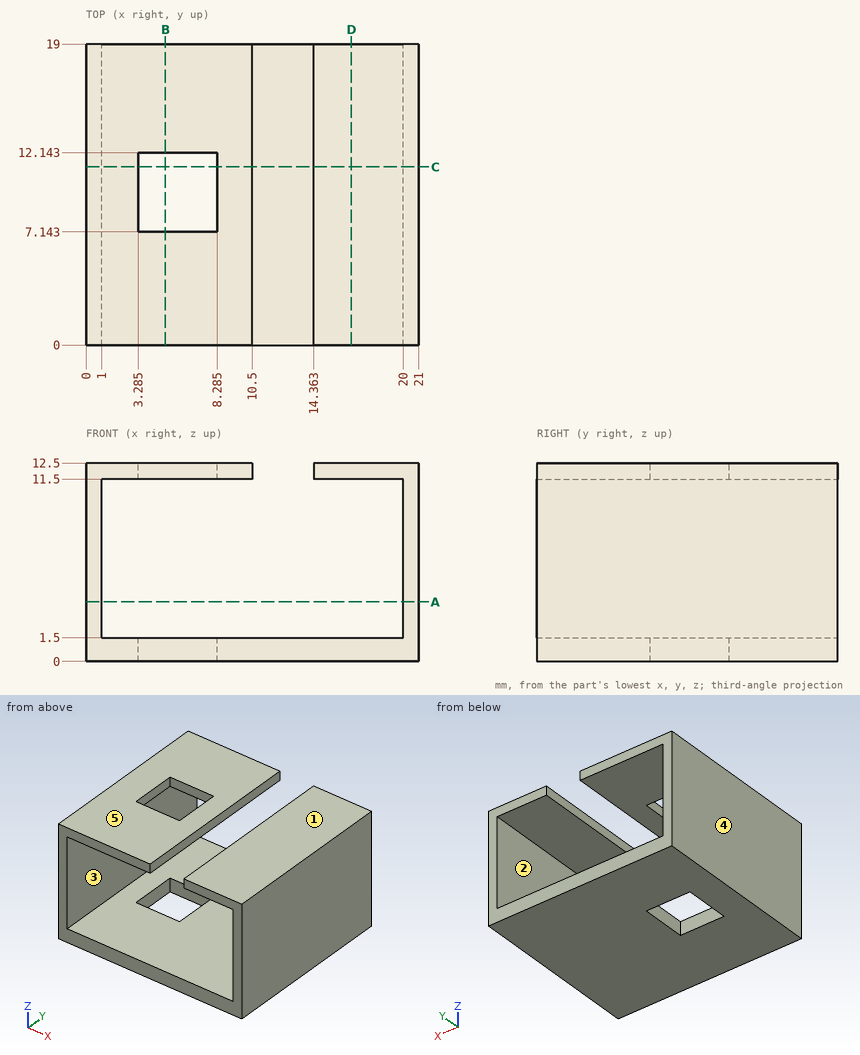
Source: three-view drawing plus pictorial views. Frame: mm from the lowest corner of the part. A direction names the side the tool comes from. Round coordinates to 2 decimals unless told otherwise and drop trailing zeros. Loops run counter-clockwise (first coordinate to the right, second up) from the corner with the lowest first, then second, coordinate; pieces in that order, holes last. Notation, with made-up numbers: M 5,44.25 L 32,44.25 A25 ccw 32,68.25 Z; hole C 58,39.25 d6. An arc over 180 degrees is marked long. Put each result on its own line as item: value. Start each with the question number.
(1) Section query D-D (x = 16.75). Return loops of the section in (y, z).
(2) Section query A-A (z = 3.75). Return loops of the section in (x, y).
(3) Section query C-C (y = 11.25). Return loops of the section in (x, z) (1 decimal).
(4) Draft query along X for the marked faces 3, 4 and 5. Return one class per face: +X half, -X half, draft (parallel to the pull), parting line (faces both ways), or undercut.
(5) Section query B-B (x = 5). Return loops of the section in (y, z).
(6) Material intervals for line 1 along Z through (x, y) = (3.25, 1.5); line 2 along X through (y, z) = (5, 4); line 3 along Y through (x, z) = (6.25, 1), sorted ascending. Write a range as [from, to].
(7) Contact query for a flat-ended pin moving along its axis: pin 1 Ø0.8 at (x, z) = (6.5, 1) entering from -Y. Output: stop coordinate, or through.
(8) Set-up query: the marked faces 1 and 2. Return all of +Z, -Z, +X, -X, +Y, -Y with unobstructed straight access to the full face (end or side cutting, diameter ignored); none if empty.
Findings below:
1. outline: M 0,0 L 19,0 L 19,1.5 L 0,1.5 Z; M 0,11.5 L 19,11.5 L 19,12.5 L 0,12.5 Z
2. outline: M 0,0 L 1,0 L 1,19 L 0,19 Z; M 20,0 L 21,0 L 21,19 L 20,19 Z
3. outline: M 0,0 L 3.3,0 L 3.3,1.5 L 1,1.5 L 1,11.5 L 3.3,11.5 L 3.3,12.5 L 0,12.5 Z; M 8.3,0 L 21,0 L 21,12.5 L 14.4,12.5 L 14.4,11.5 L 20,11.5 L 20,1.5 L 8.3,1.5 Z; M 8.3,11.5 L 10.5,11.5 L 10.5,12.5 L 8.3,12.5 Z
4. face 3: undercut
4. face 4: -X half
4. face 5: draft
5. outline: M 0,0 L 7.14,0 L 7.14,1.5 L 0,1.5 Z; M 0,11.5 L 7.14,11.5 L 7.14,12.5 L 0,12.5 Z; M 12.14,0 L 19,0 L 19,1.5 L 12.14,1.5 Z; M 12.14,11.5 L 19,11.5 L 19,12.5 L 12.14,12.5 Z
6. line 1: z = [0, 1.5], [11.5, 12.5]
6. line 2: x = [0, 1], [20, 21]
6. line 3: y = [0, 7.14], [12.14, 19]
7. pin 1: stops at y = 0
8. face 1: +Z, +X, -X, +Y, -Y
8. face 2: +Y, -Y
